Check sheet for the drawn part. Datum: minimum x, y, z corner. Units: mm. A direction names the side the tool comes from. Give positions to 0.01 mm unless a question says otherwise; leave off trailing zeros. Order: outer loops, then holes, each group sorted by start corner. A loop starts at its lowest first (then second) coordinate and runs counter-clockwise, first axis right, second up. Notation, with made-up numbers: (9, 88.25) -> (45, 88.25) arc R21 cw to (45, 111.25) -> close; hole circle Ø11 at (-35, 25). An arc over 180 degrees is marked (long way). Return JSON: item names as keys, results as strings. Group by question number.
(1) Cross-section at D-D on x = 21. Enter the section's corners in (y, z).
(2) Cross-section at A-A on z = 6. Enter the section's corners in (x, y), then the cut area to 3 significant figures.
(3) Tool access check on the marked faces 1, 2 and 3. Record the directions out of +Z, -Z, +X, -X, +Y, -Y that give a thin tool (end or side, any length) a straight path to the whole face; none if there is none.
(4) Cross-section at C-C on x = 39. Enter the section's corners in (y, z), then the cut area to 3 significant figures.
(5) Depth check by flat-ended pin: pin 1 Ø5 at (x, y) = (27, 6.5) entering from -Z; pin 2 Ø4 at (y, z) = (7, 9) entering from -X; pin 3 Ø1 at (x, z) = (75, 8.5) entering from +Y; pin 4 Ø1 at (y, z) = (10.5, 7.5) entering from -X. Enter the tip coordinate at first touch or a pass-through.
(6) Thickness scan on line 1 along X through (y, z) = (3, 8); line 2 along X through (y, z) = (10.75, 4.25); line 3 along Y through (x, z) = (34, 4.5). Record the ranges inside material, lowest first.
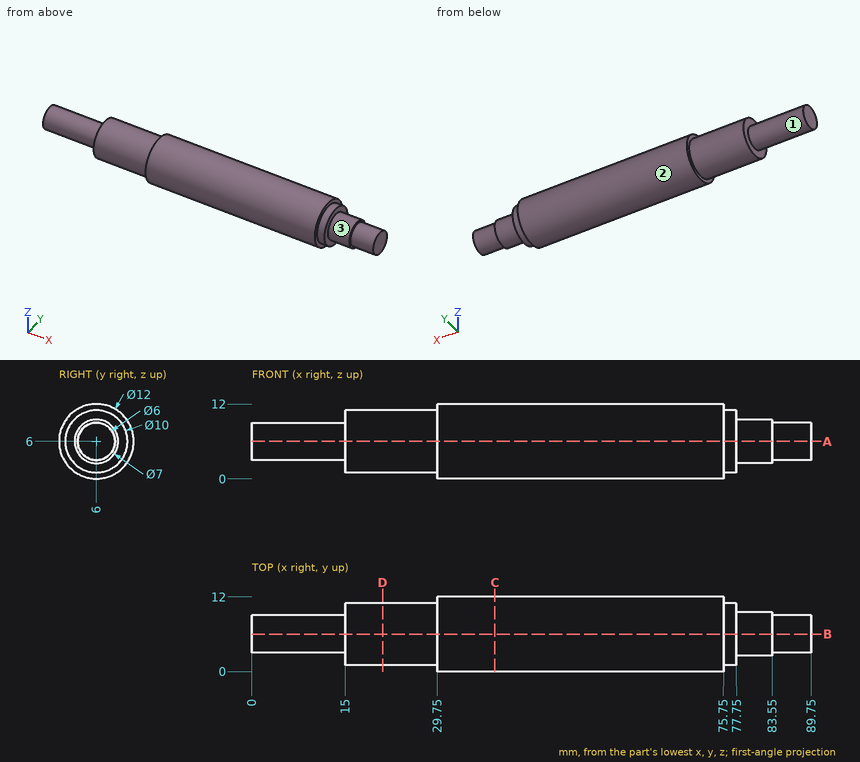
Verdict:
{
 "1": {"outline": "circle Ø10 at (6, 6)"},
 "2": {"outline": "(0, 3) -> (15, 3) -> (15, 1) -> (29.75, 1) -> (29.75, 0) -> (75.75, 0) -> (75.75, 1) -> (77.75, 1) -> (77.75, 2.5) -> (83.55, 2.5) -> (83.55, 3) -> (89.75, 3) -> (89.75, 9) -> (83.55, 9) -> (83.55, 9.5) -> (77.75, 9.5) -> (77.75, 11) -> (75.75, 11) -> (75.75, 12) -> (29.75, 12) -> (29.75, 11) -> (15, 11) -> (15, 9) -> (0, 9) -> close", "area": "887 mm²"},
 "3": {"face 1": "-X", "face 2": "+X, -X", "face 3": "+X"},
 "4": {"outline": "circle Ø12 at (6, 6)", "area": "113 mm²"},
 "5": {"pin 1": "z = 1", "pin 2": "x = 0", "pin 3": "y = 11.66", "pin 4": "x = 15"},
 "6": {"line 1": "15 to 77.75", "line 2": "29.75 to 75.75", "line 3": "0.19 to 11.81"}
}
